Can you work these out from the drawing? Everything is in mm from the part's minimum corner. A direction names the side the tool comes from. Give positions to 0.01 mm unless a question says otherwise; leave off trailing zeros. Write each loop counter-clockwise with the first axis right and the second up, starting at its lowest first coordinate (ties: lowest second). Pieces come first, ordered by that corner, then holes. Notation, with made-up numbers: (-21, -27) - (10, -27) arc R24 ccw to (10, -4) - close; hole circle Ø2 at (51.5, -31.75). An arc over 180 degrees is marked (long way). Return JSON: item names as keys, results as strings. Group by question number.
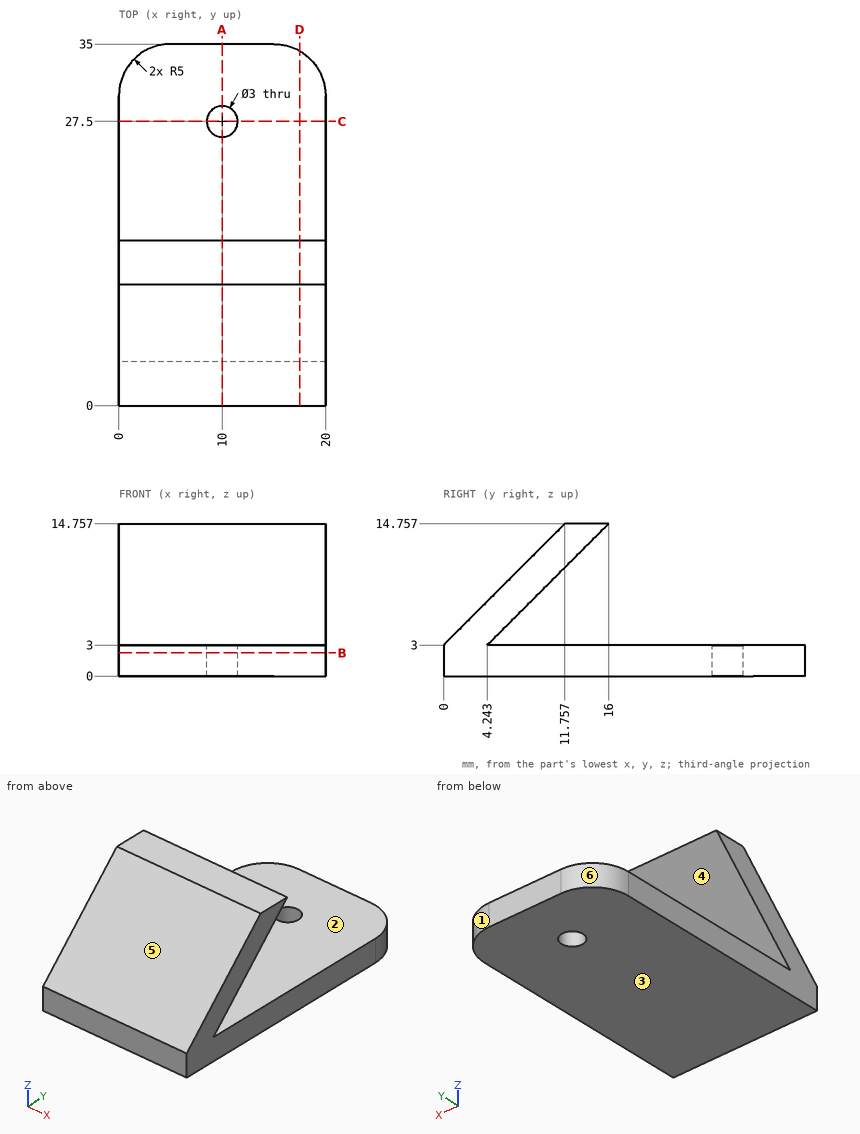
1) I need wall thicknesses on line 1 along Y through (x, z) = (10, 2); line 2 along X through (y, z) = (27.5, 2.05); line 3 along Z through (x, y) = (3.5, 17). Which ranges of each line are inside material? Lowest first, please.
2) Imagine slicing it at D-D, the plane x = 17.5. Write out the boundary of the cut face in (y, z), and give its area (3 significant figures).
3) Imagine slicing it at B-B, the plane z = 2.25. Write out the boundary of the cut face in (x, y), and give its area (3 significant figures).
4) Imagine slicing it at A-A, the plane x = 10. Write out the boundary of the cut face in (y, z), and give its area (3 significant figures).
5) On a 3-axis mill with a long thin cutter (end or side, diameter ignored), from which of +Z, -Z, +X, -X, +Y, -Y can I reach the whole of each face in a straight line? I mean the marked faces 1 and 2. Say none if no direction works.
6) Imagine slicing it at C-C, the plane y = 27.5. Write out the boundary of the cut face in (x, z), and give its area (3 significant figures).
7) Will these pins go through, and if not, where does the flat tip stop? pin 1 Ø4 at (x, z) = (6, 7) entering from -Y; pin 2 Ø1.5 at (x, z) = (11.5, 5.5) entering from +Y; pin 3 Ø1.5 at (x, z) = (2, 7.5) entering from -Y.
8) We'd pull the mould along Z, two halves only. Please class the marked faces 3, 4, 5 and 6: pulls with the +Z half, pulls with the -Z half, needs draft (parallel to the pull), parting line crosses it, or undercut.
Resolved:
{
 "1": {"line 1": "0 to 26, 29 to 35", "line 2": "0 to 8.5, 11.5 to 20", "line 3": "0 to 3"},
 "2": {"outline": "(0, 0) - (34.33, 0) - (34.33, 3) - (4.24, 3) - (16, 14.76) - (11.76, 14.76) - (0, 3) - close", "area": "153 mm^2"},
 "3": {"outline": "(0, 0) - (20, 0) - (20, 30) arc R5 ccw to (15, 35) - (5, 35) arc R5 ccw to (0, 30) - close; hole circle Ø3 at (10, 27.5)", "area": "682 mm^2"},
 "4": {"outline": "(0, 0) - (26, 0) - (26, 3) - (4.24, 3) - (16, 14.76) - (11.76, 14.76) - (0, 3) - close; (29, 0) - (35, 0) - (35, 3) - (29, 3) - close", "area": "146 mm^2"},
 "5": {"face 1": "+Z, -Z, +X, +Y", "face 2": "+X, -X, +Y"},
 "6": {"outline": "(0, 0) - (8.5, 0) - (8.5, 3) - (0, 3) - close; (11.5, 0) - (20, 0) - (20, 3) - (11.5, 3) - close", "area": "51.0 mm^2"},
 "7": {"pin 1": "y = 2", "pin 2": "y = 7.49", "pin 3": "y = 3.75"},
 "8": {"face 3": "pulls with the -Z half", "face 4": "undercut", "face 5": "pulls with the +Z half", "face 6": "needs draft"}
}
